from build123d import *

# Parameters (mm, degrees)
BOSS_EXTRUDE1_DEPTH = 9
BOSS_EXTRUDE2_DEPTH = 2.5
SKETCH5_W           = 2.5
SKETCH5_H           = 10
BOSS_EXTRUDE3_DEPTH = 3.5
BOSS_EXTRUDE4_DEPTH = 9
SKETCH7_R           = 1
CUT_EXTRUDE2_DEPTH  = 9


with BuildPart() as part:
    # Sketch1 → Boss-Extrude1 (new body)
    with BuildSketch(Plane.XY):
        Polygon((-8.689412161, 3.413307669), (-8.5, 14), (-6.5, 14), (-6.714698402, 2), (6.714698402, 2), (6.5, 14), (8.5, 14), (8.695807241, 3.055871556), (8.750481469, 0), (5.5, 0), (5.5, -6), (3.5, -6), (3.5, 0), (-3.5, 0), (-3.5, -6), (-5.5, -6), (-5.5, 0), (-8.750481469, 0), align=None)
    extrude(amount=BOSS_EXTRUDE1_DEPTH)

    # Sketch3 → Boss-Extrude2 (add)
    with BuildSketch(Plane(origin=(0, 0, 0), x_dir=(-1, 0, 0), z_dir=(0, 0, -1))):
        Polygon((-8.5, 14), (-6.5, 14), (-6.678915335, 4), (-8.678915335, 4), align=None)
        Polygon((6.5, 14), (8.5, 14), (8.678915335, 4), (6.678915335, 4), align=None)
    extrude(amount=BOSS_EXTRUDE2_DEPTH)

    # Sketch5 → Boss-Extrude3 (add)
    with BuildSketch(Plane(origin=(8.747681276, 0.156509433, 0), x_dir=(0, 0, -1), z_dir=(0.9998399849293209, 0.01788867061956491, 0))):
        with Locations((1.25, 8.845706089)):
            Rectangle(SKETCH5_W, SKETCH5_H)
    boss_extrude3 = extrude(amount=BOSS_EXTRUDE3_DEPTH)

    # Sketch6 → Boss-Extrude4 (add)
    with BuildSketch(Plane.XY):
        Polygon((10.999439947, 14.044718814), (11.999439947, 14.062610347), (12.249921417, 4.062610347), (11.249921417, 4.044718814), align=None)
    boss_extrude4 = extrude(amount=BOSS_EXTRUDE4_DEPTH)

    # Mirror2: Boss-Extrude3, Boss-Extrude4 across plane
    add(boss_extrude3.mirror(Plane(origin=(0, 0, 0), x_dir=(0, 0, 1), z_dir=(1, 0, 0))))
    add(boss_extrude4.mirror(Plane(origin=(0, 0, 0), x_dir=(0, 0, 1), z_dir=(1, 0, 0))))

    # Sketch7 → Cut-Extrude2 (cut)
    with BuildSketch(Plane(origin=(-6.748321285, 0.120737817, 0), x_dir=(0, 0, -1), z_dir=(0.9998399849293208, -0.017888670619572784, 0))):
        with Locations(Location((-3.25, 10.879562942, 0), (0, 0, 90))):
            Circle(SKETCH7_R)
    cut_extrude2 = extrude(amount=-CUT_EXTRUDE2_DEPTH, mode=Mode.SUBTRACT)

    # Mirror3: Cut-Extrude2 across plane
    add(cut_extrude2.mirror(Plane(origin=(0, 0, 0), x_dir=(0, 0, 1), z_dir=(1, 0, 0))), mode=Mode.SUBTRACT)


solid = part.part
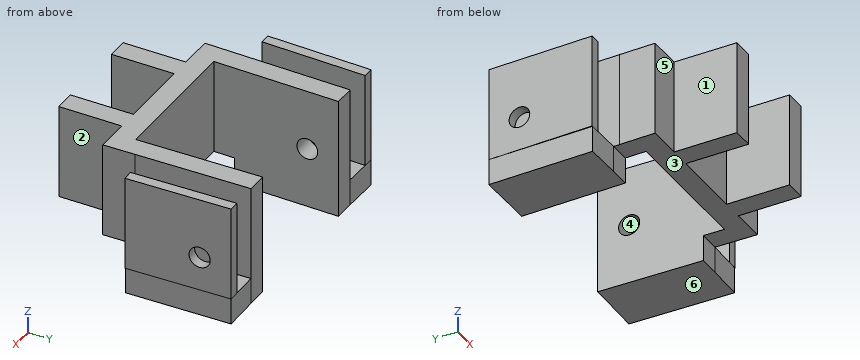
The listing builds one solid part. Answer for the finished solid, in the listing's coordinates (mm). Face numbers are marked on the shaded views. A direction names the side the tool comes from. Coordinates: 2 decimals unless noted, no trailing zeros. Loops run counter-clockwise (first coordinate to the right, second up) from the corner with the lowest first, then second, coordinate; pieces in that order, holes last. Notation, with made-up numbers: (49, 54.5) -> (101, 54.5) arc R20 ccw to (101, 69.5) -> close; hole circle Ø2 at (-18.5, 9). An arc over 180 degrees is marked (long way). Answer in a Markdown table with one row per item. Add a question column.
1. The part is cut by section D-D, the plane x = 4.5. Write down the section's boundary in (y, z), then the cut area to 3 significant figures.
2. The part is cut by section A-A, the plane z = 1. Write down the section's boundary in (x, y).
3. Consider line 1 (X direction, y = -3, z = 0.25); line 2 (X direction, y = 9, z = 7); line 3 (X direction, y = 12, z = 6.75). Determine where each line is inside the solid, lowest interval first. Write a range as [from, to].
4. For the marked faces 1, 2 and 3, determine the directions among +Z, -Z, +X, -X, +Y, -Y from which every point of the face is accessible in a straight line to the end or side of a thin tool.
5. Determine the mould class of the marked faces 4, 5 and 6 for opening direction Z: +Z half, -Z half, draft (parallel to the pull), parting line (faces both ways), or undercut.
6. Flat-ended cylindrical pins translate along their axes: P1, Ø5, axis at y = -3, z = 3.5, coming from the +X side; P2, Ø1, axis at x = -8, z = 6.5, coming from the -Y side; P3, Ø0.8, axis at x = -9.5, y = 7, coming from the +Z side; P4, Ø3, axis at x = 10.5, y = 11.5, coming from the +Z side. Find the tip coordinate at first contact, or state that the pin passes through.
7. The part is cut by section B-B, the plane y = -2.75. Write down the section's boundary in (x, z).
Answer below:
| question | item | result |
|---|---|---|
| 1 | outline | (-6, 0) -> (2, 0) -> (2, 9) -> (-6, 9) -> close |
| 1 | area | 72.0 mm2 |
| 2 | outline | (-12.25, 4.06) -> (-11.25, 4.04) -> (-11, 14.04) -> (-12, 14.06) -> close; (-8.75, 0) -> (-5.5, 0) -> (-5.5, -6) -> (-3.5, -6) -> (-3.5, 0) -> (3.5, 0) -> (3.5, -6) -> (5.5, -6) -> (5.5, 0) -> (8.75, 0) -> (8.5, 14) -> (6.5, 14) -> (6.71, 2) -> (-6.71, 2) -> (-6.5, 14) -> (-8.5, 14) -> close; (11, 14.04) -> (11.25, 4.04) -> (12.25, 4.06) -> (12, 14.06) -> close |
| 3 | line 1 | [-5.5, -3.5], [3.5, 5.5] |
| 3 | line 2 | [-12.13, -11.13], [-8.59, -6.59], [6.59, 8.59], [11.13, 12.13] |
| 3 | line 3 | [-12.05, -11.05], [-8.54, -6.54], [6.54, 8.54], [11.05, 12.05] |
| 4 | face 1 | +Z, -Z, -X, -Y |
| 4 | face 2 | +Z, -Z, +X, -Y |
| 4 | face 3 | -Z, +X, -X, -Y |
| 5 | face 4 | undercut |
| 5 | face 5 | draft |
| 5 | face 6 | -Z half |
| 6 | P1 | x = 5.5 |
| 6 | P2 | y = 0 |
| 6 | P3 | z = 0 |
| 6 | P4 | z = 9 |
| 7 | outline | (-5.5, 0) -> (-3.5, 0) -> (-3.5, 9) -> (-5.5, 9) -> close; (3.5, 0) -> (5.5, 0) -> (5.5, 9) -> (3.5, 9) -> close |
